Work out the finished part from the listing and answer in its coordinate system (mm). A direction names the side the tool comes from. Coordinates: 2 decimals unless noted, no trailing zeros. Loops run counter-clockwise (first coordinate to the right, second up) from the corner with the lowest first, then second, coordinate; pieces in that order, holes last. Notation, with made-up numbers: (-8, 23) - (48, 23) arc R12 cw to (48, 27) - close; hole circle Ø1 at (88, 46). An arc over 180 degrees is marked (long way). Write each question's results on one line, items separated by ' | '. Start each with the question number.
1. A cutting plane is placed at C-C on x = -69. Determine the outline of the cut face in (y, z), then the cut area to 3 significant figures.
2. A cutting plane is placed at A-A on y = -13.5. Determine the outline of the cut face in (x, z), then the cut area to 3 significant figures.
3. Determine the mould class of faces 5 (the flat face through (-101, 1, 0)), 6 (the flat face through (0, 100, 24)), 7 (the flat face through (-6, -90, 25)), 8 (the flat face through (95, 19, 25)) for opening direction Y: released by +Y, released by -Y, zero draft, split by the parting line, or undercut.
4. Each of these flat-tipped pins is pushed along its axis until it touches: P1, Ø3, axis at x = -6, z = 24.54, coming from the -Y side; P2, Ø1, axis at x = -12, y = -27.5, coming from the -Z side. Where does it stop, or does it pass through?
5. Which of the six approach directions +Z, -Z, +X, -X, +Y, -Y give full straight-line access (tool end or side, diameter ignored) to faces 1 (the cylindrical face through (12.48, -95.07, 26.53)), 2 (the flat face through (-97, 95, 10)), 3 (the flat face through (-3, 90, 25)), 4 (the flat face through (-105, -1, 15))?
6. A cutting plane is placed at B-B on z = 7.5. Determine the outline of the cut face in (x, y), then the cut area to 3 significant figures.
7. Find the intervals of material crossed by line 1 along Y through (x, z) = (-37, 24); line 2 along X through (y, z) = (67, 22); line 3 along X through (y, z) = (-69.5, 15.25), in increasing order. Write a range as [from, to].
from build123d import *

# Parameters (mm, degrees)
SKETCH1_W           = 210
SKETCH1_H           = 200
BOSS_EXTRUDE1_DEPTH = 30
SKETCH2_W           = 194
SKETCH2_H           = 20
CUT_EXTRUDE1_DEPTH  = 228.870577302
CUT_EXTRUDE2_DEPTH  = 149.07092895
CUT_EXTRUDE3_DEPTH  = 149.07092895
SKETCH5_R           = 2.5
CUT_EXTRUDE4_DEPTH  = 10


with BuildPart() as part:
    # Sketch1 → Boss-Extrude1 (new body)
    with BuildSketch(Plane.XY):
        Rectangle(SKETCH1_W, SKETCH1_H)
    extrude(amount=BOSS_EXTRUDE1_DEPTH)

    # Sketch2 → Cut-Extrude1 (cut, through all)
    with BuildSketch(Plane(origin=(0, -100, 0), x_dir=(-1, 0, 0), z_dir=(0, -1, 0))):
        with Locations((0, -10)):
            Rectangle(SKETCH2_W, SKETCH2_H)
    extrude(amount=-CUT_EXTRUDE1_DEPTH, mode=Mode.SUBTRACT)

    # Sketch3 → Cut-Extrude2 (cut, through all)
    with BuildSketch(Plane.XY.offset(30)):
        with BuildLine():
            Line((88, 85), (88, -45))
            ThreePointArc((88, -45), (91.5, -48.5), (95, -45))
            Line((95, -45), (95, 85))
            ThreePointArc((95, 85), (91.5, 88.5), (88, 85))
        make_face()
    extrude(amount=-CUT_EXTRUDE2_DEPTH, mode=Mode.SUBTRACT)

    # Sketch4 → Cut-Extrude3 (cut, through all)
    with BuildSketch(Plane.XY.offset(30)):
        with BuildLine():
            Line((91.5, 83), (-95, 83))
            ThreePointArc((-95, 83), (-98.5, 86.5), (-95, 90))
            Line((-95, 90), (91.5, 90))
            ThreePointArc((91.5, 90), (95, 86.5), (91.5, 83))
        make_face()
    extrude(amount=-CUT_EXTRUDE3_DEPTH, mode=Mode.SUBTRACT)

    # Sketch5 → Cut-Extrude4 (cut)
    with BuildSketch(Plane.XZ.offset(100)):
        with Locations(Location((-6, 24.544570078, 0), (0, 0, 270))):
            Circle(SKETCH5_R)
        with Locations(Location((14, 24.544570078, 0), (0, 0, 270))):
            Circle(SKETCH5_R)
    extrude(amount=-CUT_EXTRUDE4_DEPTH, mode=Mode.SUBTRACT)


solid = part.part
Values:
1) outline: (-100, 20) - (83, 20) - (83, 30) - (-100, 30) - close; (90, 20) - (100, 20) - (100, 30) - (90, 30) - close | area: 1,930 mm^2
2) outline: (-105, 0) - (-97, 0) - (-97, 20) - (88, 20) - (88, 30) - (-105, 30) - close; (95, 20) - (97, 20) - (97, 0) - (105, 0) - (105, 30) - (95, 30) - close | area: 2,350 mm^2
3) face 5: zero draft | face 6: released by +Y | face 7: released by -Y | face 8: undercut
4) P1: y = -90 | P2: z = 20
5) face 1: -Y | face 2: -Z, +Y, -Y | face 3: +Z, -Z | face 4: +Z, -Z, -X, +Y, -Y
6) outline: (-105, -100) - (-97, -100) - (-97, 83.63) arc R3.5 cw to (-97, 89.37) - (-97, 100) - (-105, 100) - close; (97, -100) - (105, -100) - (105, 100) - (97, 100) - close | area: 3,190 mm^2
7) line 1: [-100, 83], [90, 100] | line 2: [-105, 88], [95, 105] | line 3: [-105, -97], [97, 105]
